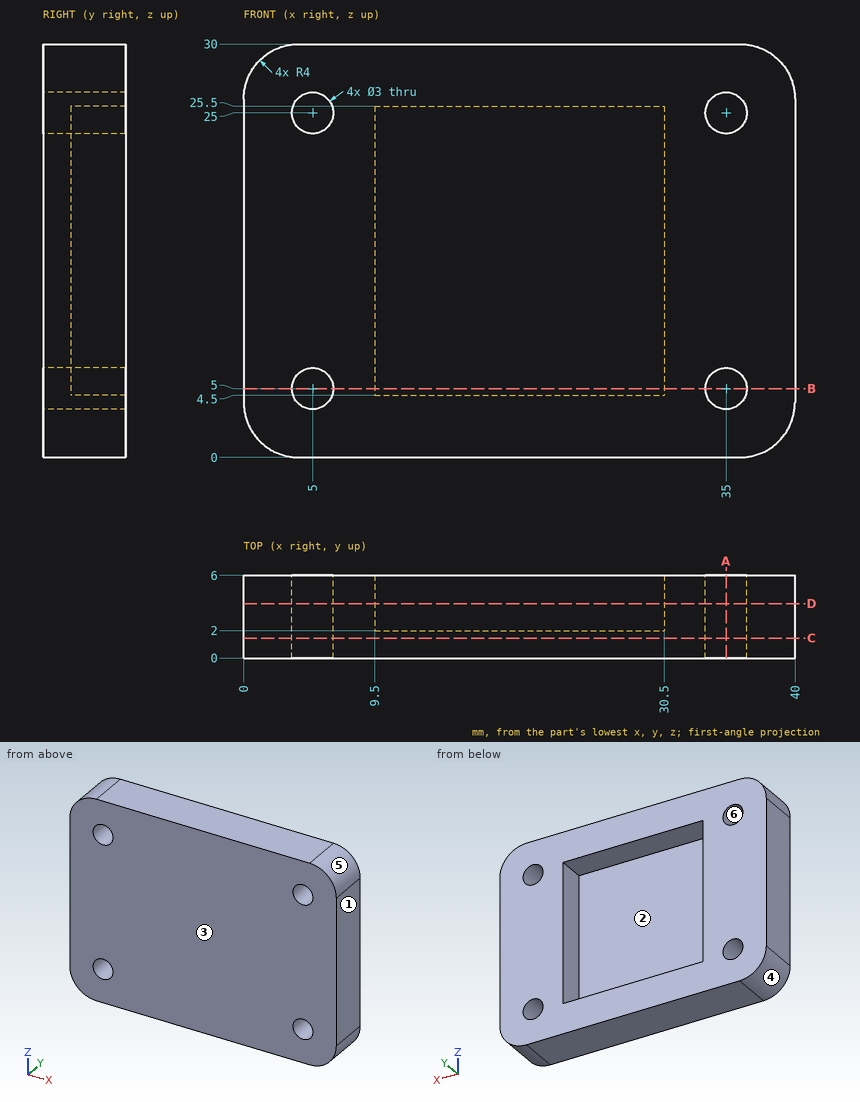
Answer from the drawing. Dimensions are ordinates in mm from the lowest x, y and z of the part. A direction names the side the tool comes from. Give positions to 0.01 mm unless a question says otherwise; leave off trailing zeros. Loops run counter-clockwise (first coordinate to the right, second up) from the corner with the lowest first, then second, coordinate; pieces in that order, holes last. Notation, with made-up numbers: M 87,39 L 142,39 A24 ccw 142,60 Z; hole C -28,-8.5 d2. An arc over 180 degrees is marked long. One line per item, written item: value.
Q1. For the marked faces 1 and 2, determine the directions among +Z, -Z, +X, -X, +Y, -Y from which every point of the face is accessible in a straight line to the end or side of a thin tool.
Working result:
face 1: +Z, -Z, +X, +Y, -Y
face 2: +Y
Q2. A cutting plane is placed at B-B on z = 5. Determine the outline of the cut face in (x, y).
Working result:
outline: M 0,0 L 3.5,0 L 3.5,6 L 0,6 Z; M 6.5,0 L 33.5,0 L 33.5,6 L 30.5,6 L 30.5,2 L 9.5,2 L 9.5,6 L 6.5,6 Z; M 36.5,0 L 40,0 L 40,6 L 36.5,6 Z
Q3. A cutting plane is placed at C-C on y = 1.45. Determine the outline of the cut face in (x, z).
Working result:
outline: M 0,4 A4 ccw 4,0 L 36,0 A4 ccw 40,4 L 40,26 A4 ccw 36,30 L 4,30 A4 ccw 0,26 Z; hole C 5,5 d3; hole C 5,25 d3; hole C 35,5 d3; hole C 35,25 d3
Q4. A cutting plane is placed at A-A on x = 35. Determine the outline of the cut face in (y, z).
Working result:
outline: M 0,0 L 6,0 L 6,3.5 L 0,3.5 Z; M 0,6.5 L 6,6.5 L 6,23.5 L 0,23.5 Z; M 0,26.5 L 6,26.5 L 6,30 L 0,30 Z
Q5. A flat-ended cylindrical pin translates along its axis: P1, Ø17, axis at x = 16.5, z = 18, coming from the +Y side. Find the tip coordinate at first contact, or state that the pin passes through.
Working result:
P1: stops at y = 6
Q6. A cutting plane is placed at D-D on y = 3.95. Determine the outline of the cut face in (x, z), then the cut area to 3 significant figures.
Working result:
outline: M 0,4 A4 ccw 4,0 L 36,0 A4 ccw 40,4 L 40,26 A4 ccw 36,30 L 4,30 A4 ccw 0,26 Z; hole C 5,5 d3; hole C 5,25 d3; hole M 9.5,4.5 L 30.5,4.5 L 30.5,25.5 L 9.5,25.5 Z; hole C 35,5 d3; hole C 35,25 d3
area: 717 mm^2
Q7. Determine the mould class of the marked faces 3, 4, 5 and 6 for opening direction Z: +Z half, -Z half, draft (parallel to the pull), parting line (faces both ways), or undercut.
Working result:
face 3: draft
face 4: -Z half
face 5: +Z half
face 6: undercut
Q8. Find the intervals of material crossed by line 1 (X direction, y = 1.9, z = 25); line 2 (X direction, y = 3.65, z = 5); line 3 (X direction, y = 3.35, z = 16.5), in increasing order. Write a range as from..to.
Working result:
line 1: x = 0..3.5, 6.5..33.5, 36.5..40
line 2: x = 0..3.5, 6.5..9.5, 30.5..33.5, 36.5..40
line 3: x = 0..9.5, 30.5..40
